```python
from build123d import *

# Parameters (mm, degrees)
SKETCH_1_W      = 23.1
SKETCH_1_H      = 25.5
SKETCH_1_R      = 0.9
EXTRUDE_1_DEPTH = 1.2
SKETCH_2_W      = 15
SKETCH_2_H      = 16
EXTRUDE_2_DEPTH = 4
SKETCH_3_R      = 5.5
EXTRUDE_3_DEPTH = 0.2
SKETCH_4_W      = 10.4
SKETCH_4_H      = 4.9
EXTRUDE_4_DEPTH = 3
SKETCH_5_W      = 7.083649358
SKETCH_5_H      = 16.349953635
SKETCH_5_W_2    = 1.366011138
SKETCH_5_H_2    = 2.325890212
SKETCH_5_W_3    = 1.835080991
SKETCH_5_H_3    = 1.91855554
SKETCH_5_W_4    = 3.175010274
SKETCH_5_H_4    = 13.27010499
SKETCH_5_W_5    = 4.111087422
SKETCH_5_H_5    = 2.03375188
SKETCH_5_W_6    = 5.947363934
SKETCH_5_H_6    = 10.708861721
EXTRUDE_5_DEPTH = 0.8


with BuildPart() as part:
    # 草图1 → 凸台-拉伸1 (new body)
    with BuildSketch(Plane(origin=(0, 0, 0), x_dir=(1, 0, 0), z_dir=(0, 1, 0))):
        Rectangle(SKETCH_1_W, SKETCH_1_H)
        with Locations((10, 11.15)):
            Circle(SKETCH_1_R, mode=Mode.SUBTRACT)
        with Locations((-10, 11.15)):
            Circle(SKETCH_1_R, mode=Mode.SUBTRACT)
        with Locations((10, -11.15)):
            Circle(SKETCH_1_R, mode=Mode.SUBTRACT)
        with Locations((-10, -11.15)):
            Circle(SKETCH_1_R, mode=Mode.SUBTRACT)
    extrude(amount=EXTRUDE_1_DEPTH)

    # 草图2 → 凸台-拉伸2 (add)
    with BuildSketch(Plane(origin=(0, 1.2, 0), x_dir=(1, 0, 0), z_dir=(0, 1, 0))):
        with Locations((0, 2.75)):
            Rectangle(SKETCH_2_W, SKETCH_2_H)
    extrude(amount=EXTRUDE_2_DEPTH)

    # 草图3 → 凸台-拉伸3 (add)
    with BuildSketch(Plane(origin=(0, 5.2, 0), x_dir=(1, 0, 0), z_dir=(0, 1, 0))):
        with Locations((0, 2.25)):
            Circle(SKETCH_3_R)
    extrude(amount=EXTRUDE_3_DEPTH)

    # 草图4 → 凸台-拉伸4 (add)
    with BuildSketch(Plane(origin=(0, 1.2, 0), x_dir=(1, 0, 0), z_dir=(0, 1, 0))):
        with Locations((0, -10.2)):
            Rectangle(SKETCH_4_W, SKETCH_4_H)
    extrude(amount=EXTRUDE_4_DEPTH)

    # 草图5 → 凸台-拉伸5 (add)
    with BuildSketch(Plane.XZ):
        with Locations((-0.031355778, 3.113299148)):
            Rectangle(SKETCH_5_W, SKETCH_5_H)
        with Locations((-3.127935708, -7.143071696)):
            Rectangle(SKETCH_5_W_2, SKETCH_5_H_2)
        with Locations((7.782140552, -3.170898119)):
            Rectangle(SKETCH_5_W_3, SKETCH_5_H_3)
        with Locations((-7.914690991, 2.157353718)):
            Rectangle(SKETCH_5_W_4, SKETCH_5_H_4)
        with Locations((-8.028697172, -7.143071696)):
            Rectangle(SKETCH_5_W_5, SKETCH_5_H_5)
        with Locations((7.909232795, 3.891185517)):
            Rectangle(SKETCH_5_W_6, SKETCH_5_H_6)
    extrude(amount=EXTRUDE_5_DEPTH)


solid = part.part
```
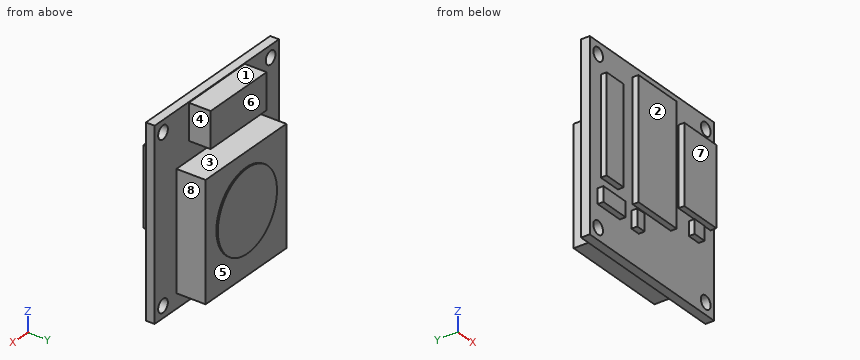
Geometry: final body of the model. Coordinates: model frame, mm. Face numbers are marked on the shaded views. A direction names the side the tool comes from. Round coordinates to 2 decimals unless told otherwise and drop trailing zeros. Loops run counter-clockwise (first coordinate to the right, second up) from the corner with the lowest first, then second, coordinate; pieces in that order, holes last.
Item 1: Section C-C, the plane y = 0.5. Output: boundary loops of the cut face in (x, z).
Checked values:
outline: (-11.55, -12.75) - (11.55, -12.75) - (11.55, 12.75) - (-11.55, 12.75) - close; hole circle Ø1.8 at (-10, -11.15); hole circle Ø1.8 at (-10, 11.15); hole circle Ø1.8 at (10, -11.15); hole circle Ø1.8 at (10, 11.15)
Item 2: Section A-A, the plane x = 10. Output: boundary loops of the cut face in (y, z), plus the area to 3 significant figures.
Checked values:
outline: (-0.8, -1.46) - (0, -1.46) - (0, -10.25) - (1.2, -10.25) - (1.2, 10.25) - (0, 10.25) - (0, 9.25) - (-0.8, 9.25) - close; (0, -12.75) - (1.2, -12.75) - (1.2, -12.05) - (0, -12.05) - close; (0, 12.05) - (1.2, 12.05) - (1.2, 12.75) - (0, 12.75) - close
area: 34.8 mm2
Item 3: Contact query for flat-ended pins moving along their axis: P1, Ø3, axis at x = -6.5, z = 6.5, coming from the +Y side; P2, Ø0.6, axis at y = -0.5, z = -6.5, coming from the -X side; P3, Ø0.9, axis at y = -0.5, z = -3.5, coming from the -X side; P4, Ø1.6, axis at x = 10, z = -11.15, coming from the -Y side. Output: stop coordinate, or through.
Checked values:
P1: stops at y = 5.2
P2: stops at x = -10.08
P3: stops at x = -9.5
P4: passes through
Item 4: Mould query, pull axis Z, two halves, no side actions, for the marked faces 1, 2 and 3. Classes: released by +Z, released by -Z, zero draft, split by the parting line, or undercut.
Checked values:
face 1: released by +Z
face 2: zero draft
face 3: undercut
Item 5: Line query: L1, parallel to X at y = 0.95, z = -11.15; L2, parallel to Z at x = -10, y = 0.4; L3, parallel to Z at x = 3.5, y = 1.5. Output: solid intervals per line, ascending.
Checked values:
L1: x = -11.55 to -10.9, -9.1 to 9.1, 10.9 to 11.55
L2: z = -12.75 to -12.05, -10.25 to 10.25, 12.05 to 12.75
L3: z = -10.75 to 5.25, 7.75 to 12.65
Item 6: Section D-D, the plane x = -8.5. Output: boundary loops of the cut face in (y, z).
Checked values:
outline: (-0.8, -8.16) - (0, -8.16) - (0, -12.75) - (1.2, -12.75) - (1.2, 12.75) - (0, 12.75) - (0, 8.79) - (-0.8, 8.79) - (-0.8, -4.48) - (0, -4.48) - (0, -6.13) - (-0.8, -6.13) - close
Item 7: Reachability of the marked faces 4, 5, 6, 7 and 8 from +Z, -Z, +X, -X, +Y, -Y: full face, straight path, thin tool, end or side. Return the list, or none.
Checked values:
face 4: +Z, +X, +Y
face 5: +Y
face 6: +Z, +X, -X, +Y
face 7: +Z, -Z, +X, -X, -Y
face 8: +Z, -Z, +X, +Y
Item 8: Section B-B, the plane z = -11.15. Output: boundary loops of the cut face in (x, y).
Checked values:
outline: (-11.55, 0) - (-10.9, 0) - (-10.9, 1.2) - (-11.55, 1.2) - close; (-9.1, 0) - (9.1, 0) - (9.1, 1.2) - (-9.1, 1.2) - close; (10.9, 0) - (11.55, 0) - (11.55, 1.2) - (10.9, 1.2) - close
